from build123d import *

# Parameters (mm, degrees)
BOSS_EXTRUDE1_DEPTH = 6
SKETCH2_R           = 2
CUT_EXTRUDE1_DEPTH  = 10
SKETCH3_W           = 6
SKETCH3_H           = 120
BOSS_EXTRUDE2_DEPTH = 5
SKETCH4_W           = 6
SKETCH4_H           = 10
CUT_EXTRUDE2_DEPTH  = 6
SKETCH5_W           = 42.2
SKETCH5_H           = 6
CUT_EXTRUDE3_DEPTH  = 7


with BuildPart() as part:
    # Sketch1 → Boss-Extrude1 (new body)
    with BuildSketch(Plane(origin=(0, 0, 0), x_dir=(0, 0, -1), z_dir=(1, 0, 0))):
        Polygon((39.75, 15), (39.75, 9), (-39.75, 9), (-39.75, 15), (-60, 15), (-60, -15), (60, -15), (60, 15), align=None)
    extrude(amount=BOSS_EXTRUDE1_DEPTH)

    # Sketch2 → Cut-Extrude1 (cut)
    with BuildSketch(Plane(origin=(6, 0, 0), x_dir=(0, 0, -1), z_dir=(1, 0, 0))):
        with Locations((-49.875, 0)):
            Circle(SKETCH2_R)
        with Locations((49.875, 0)):
            Circle(SKETCH2_R)
    extrude(amount=-CUT_EXTRUDE1_DEPTH, mode=Mode.SUBTRACT)

    # Sketch3 → Boss-Extrude2 (add)
    with BuildSketch(Plane(origin=(0, 15, 0), x_dir=(1, 0, 0), z_dir=(0, 1, 0))):
        with Locations((3, 0)):
            Rectangle(SKETCH3_W, SKETCH3_H)
    extrude(amount=BOSS_EXTRUDE2_DEPTH)

    # Sketch4 → Cut-Extrude2 (cut)
    with BuildSketch(Plane(origin=(6, 0, 0), x_dir=(0, 0, -1), z_dir=(1, 0, 0))):
        with Locations((-24.1, -10)):
            Rectangle(SKETCH4_W, SKETCH4_H)
        with Locations((24.1, -10)):
            Rectangle(SKETCH4_W, SKETCH4_H)
    extrude(amount=-CUT_EXTRUDE2_DEPTH, mode=Mode.SUBTRACT)

    # Sketch5 → Cut-Extrude3 (cut, through all)
    with BuildSketch(Plane(origin=(6, 0, 0), x_dir=(0, 0, -1), z_dir=(1, 0, 0))):
        with Locations((0, 6)):
            Rectangle(SKETCH5_W, SKETCH5_H)
    extrude(amount=-CUT_EXTRUDE3_DEPTH, mode=Mode.SUBTRACT)


solid = part.part
Build history of the part. All positions in model axes, mm. A direction names the side the tool comes from. Round coordinates to 2 decimals unless told otherwise and drop trailing zeros. Write each loop counter-clockwise with the first axis right and the second up, starting at its lowest first coordinate (ties: lowest second). Pieces come first, ordered by that corner, then holes. Notation, with made-up numbers: M 88.5,-5.5 L 145.5,-5.5 A18 cw 145.5,0.5 Z; hole C 75.25,-32.75 d3. An arc over 180 degrees is marked long. Answer as a JSON object with one key per item and string values. Group by question number.
(1) Cut at B-B (y = 5.5). Give the cut face in (x, z), and give its area (3 significant figures).
(2) Mould opens along Y. For faces 4 (the flat face through (3, -15, -43)), 5 (the flat face through (3, 12, -39.75)), 6 (the flat face through (3, -10, -27.1)) say: pulls with the +Y half, pulls with the -Y half, needs draft (parallel to the pull), parting line crosses it, or undercut.
(3) Cut at A-A (z = -16). Give the cut face in (x, y), and give its area (3 significant figures).
(4) Drill centre lines: L1, parallel to Y at x = 2.95, z = -34; L2, parallel to Y at x = 0.4, z = -22.5; L3, parallel to Z at x = 2.9, y = -8.5. Where is each one in solid material? Low to high.
(5) Flat gauge pins, fed straight in: pin 1 (4 mm diameter, centred on y = 11.5, z = -32, fed in from -X); pin 2 (3 mm diameter, centred on x = 4, z = -24, fed in from -Y). Where does each tip first touch, or does it go through?
(6) Cut at C-C (y = 0). Give the cut face in (x, z) (3 decimals).
(7) Which spindle directions (+Z, -Z, +X, -X, +Y, -Y) get a long thin tool onto all of the face, cutting with end or side? Do faces 1 (the flat face through (3, 2, 60)), 2 (the flat face through (3, 12, 39.75)), 3 (the flat face through (3, -5, 24)). Say none if no direction does.
(8) Cut at D-D (x = 2.35). Give the cut face in (y, z) (3 decimals).
Responses:
{
 "1": {"outline": "M 0,-60 L 6,-60 L 6,-21.1 L 0,-21.1 Z; M 0,21.1 L 6,21.1 L 6,60 L 0,60 Z", "area": "467 mm2"},
 "2": {"face 4": "pulls with the -Y half", "face 5": "undercut", "face 6": "needs draft"},
 "3": {"outline": "M 0,-15 L 6,-15 L 6,3 L 0,3 Z; M 0,15 L 6,15 L 6,20 L 0,20 Z", "area": "138 mm2"},
 "4": {"L1": "y = -15 to 9, 15 to 20", "L2": "y = -5 to 9, 15 to 20", "L3": "z = -60 to -27.1, -21.1 to 21.1, 27.1 to 60"},
 "5": {"pin 1": "passes through", "pin 2": "stops at y = -5"},
 "6": {"outline": "M 0,-60 L 6,-60 L 6,-51.875 L 0,-51.875 Z; M 0,-47.875 L 6,-47.875 L 6,47.875 L 0,47.875 Z; M 0,51.875 L 6,51.875 L 6,60 L 0,60 Z"},
 "7": {"face 1": "+Z, +X, -X, +Y, -Y", "face 2": "+X, -X", "face 3": "+X, -X, -Y"},
 "8": {"outline": "M -15,-60 L 20,-60 L 20,60 L -15,60 L -15,27.1 L -5,27.1 L -5,21.1 L -15,21.1 L -15,-21.1 L -5,-21.1 L -5,-27.1 L -15,-27.1 Z; hole C 0,-49.875 d4; hole C 0,49.875 d4; hole M 3,-21.1 L 9,-21.1 L 9,-39.75 L 15,-39.75 L 15,39.75 L 9,39.75 L 9,21.1 L 3,21.1 Z"}
}
